For this review, take the finished solid that the model builds, in its own axes (mm). Coordinates: 2 decimals unless noted, no trailing zeros. Order: outer loops, then holes, each group sorted by start corner. A loop starts at its lowest first (then second) coordinate and runs counter-clockwise, first axis right, second up. Notation, with made-up numbers: (-8, 80) -> (49, 80) arc R33 cw to (49, 108) -> close; hole circle Ø1 at (-36, -7.5). An arc over 180 degrees is marked (long way). Write item = value, one per line. Start each with the question number.
1) Consider section B-B on z = 42.5. Give the boundary of the cut face in (x, y).
2) Wall thickness on probe 1 along Y at (x, z) = (17, 35); probe 2 along Z at (x, y) = (6, 0); probe 3 along Y at (x, z) = (-32.5, 40): over which ranges is each line inside the solid? List them lowest first. Write a range as [from, to].
3) Insertion check: pin 1 Ø5 at (y, z) = (70, 35) entering from +X; pin 2 Ø3 at (y, z) = (38.5, 23.5) entering from -X; pin 3 Ø12 at (x, z) = (-99.5, 51) entering from -Y. Each pin has a flat end and moves straight along its axis. Give the tip position at first contact, or say it passes through.
4) Consider section C-C on x = -121. Give the boundary of the cut face in (y, z), and give its area (3 significant figures).
5) Consider section D-D on y = 77.5. Give the boundary of the cut face in (x, z).
6) Consider section A-A on y = 35. Give the boundary of the cut face in (x, z), and give its area (3 significant figures).
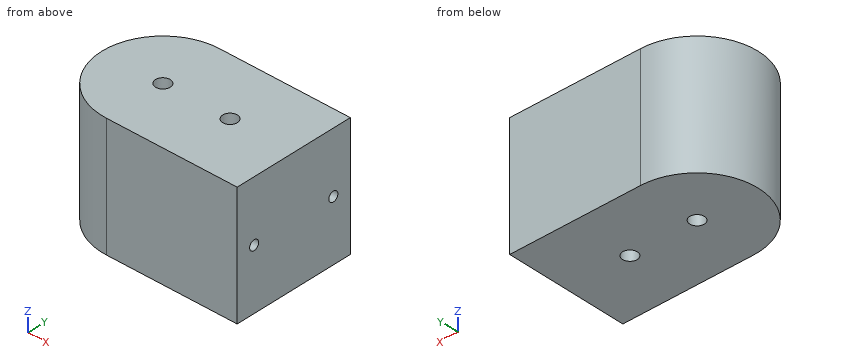
from build123d import *

# Parameters (mm, degrees)
BOSS_EXTRUDE1_DEPTH       = 70
SCALE1_SCALE              = 1.428571429
F_12_0MM_DOWEL_HOLE1_D    = 12
F_8_0MM_DOWEL_HOLE3_D     = 8
F_8_0MM_DOWEL_HOLE3_DEPTH = 20
F_8_0MM_DOWEL_HOLE3_TIP   = 2.403442476


with BuildPart() as part:
    # Sketch1 → Boss-Extrude1 (new body)
    with BuildSketch(Plane.XY):
        with BuildLine():
            Line((0, 0), (-75, 0))
            ThreePointArc((-75, 0), (-110, 35), (-75, 70))
            Line((-75, 70), (0, 70))
            Line((0, 70), (0, 0))
        make_face()
    extrude(amount=BOSS_EXTRUDE1_DEPTH)


with BuildPart() as part_1:
    # Scale1: scaled about (-51.542183312, 35, 35)
    add(part.part.scale(SCALE1_SCALE).moved(Location((22.089507134, -15, -15))))

    # Ø12.0mm Dowel Hole1 (through all)
    with Locations(Plane(origin=(-30.053350009, 35, -15), x_dir=(-1, 0, 0), z_dir=(0, 0, -1))):
        with Locations((0, 0), (55, 0)):
            Hole(F_12_0MM_DOWEL_HOLE1_D / 2)

    # Ø8.0mm Dowel Hole3
    with Locations(Plane(origin=(22.089507134, 0, 0), x_dir=(0, 0, -1), z_dir=(1, 0, 0))):
        with Locations((-35, 70), (-35, 0)):
            Hole(F_8_0MM_DOWEL_HOLE3_D / 2, depth=F_8_0MM_DOWEL_HOLE3_DEPTH)
            with Locations((0, 0, -(F_8_0MM_DOWEL_HOLE3_DEPTH + F_8_0MM_DOWEL_HOLE3_TIP / 2))):  # 118° drill point
                Cone(0, F_8_0MM_DOWEL_HOLE3_D / 2, F_8_0MM_DOWEL_HOLE3_TIP, mode=Mode.SUBTRACT)


solid = part_1.part
Answer sheet:
q1.outline = (-85.05, -15) -> (22.09, -15) -> (22.09, 85) -> (-85.05, 85) arc R50 ccw to start; hole circle Ø12 at (-85.05, 35); hole circle Ø12 at (-30.05, 35)
q2.probe_1 = [-15, -4], [4, 66], [74, 85]
q2.probe_2 = [-15, 31], [39, 85]
q2.probe_3 = [-15, 29.52], [40.48, 85]
q3.pin_1 = 1.19
q3.pin_2 = -135.01
q3.pin_3 = -14.28
q4.outline = (0.25, -15) -> (69.75, -15) -> (69.75, 85) -> (0.25, 85) -> close
q4.area = 6,950 mm2
q5.outline = (-111.39, -15) -> (22.09, -15) -> (22.09, 85) -> (-111.39, 85) -> close
q6.outline = (-135.05, -15) -> (-91.05, -15) -> (-91.05, 85) -> (-135.05, 85) -> close; (-79.05, -15) -> (-36.05, -15) -> (-36.05, 85) -> (-79.05, 85) -> close; (-24.05, -15) -> (22.09, -15) -> (22.09, 85) -> (-24.05, 85) -> close
q6.area = 13,300 mm2
